from build123d import *

# Parameters (mm, degrees)
SKETCH1_R           = 1.75
SKETCH1_R_2         = 11.5
BOSS_EXTRUDE1_DEPTH = 3.2
BOSS_EXTRUDE2_START = 3.2
SKETCH1_5_R         = 2.55
SKETCH1_5_R_2       = 3
SKETCH1_5_R_3       = 11.5
SKETCH1_5_R_4       = 1.75
BOSS_EXTRUDE2_DEPTH = 3
BOSS_EXTRUDE3_START = 5
SKETCH1_6_R         = 2.55
BOSS_EXTRUDE3_DEPTH = 1.2
CUT_EXTRUDE2_START  = 3.2
SKETCH1_4_R         = 3
CUT_EXTRUDE2_DEPTH  = 3
FILLET1_R           = 3


with BuildPart() as part:
    # Sketch1 → Boss-Extrude1 (new body)
    with BuildSketch(Plane(origin=(0, -68.726755499, 0), x_dir=(1, 0, 0), z_dir=(0, 1, 0))):
        with BuildLine():
            Line((137.12924475, -27.521572875), (137.12924475, 3.821572875))
            ThreePointArc((137.12924475, 3.821572875), (136.992227909, 4.510403054), (136.602036956, 5.094365081))
            Line((136.602036956, 5.094365081), (133.273609831, 8.422792206))
            ThreePointArc((133.273609831, 8.422792206), (132.689647804, 8.812983159), (132.000817625, 8.95))
            Line((132.000817625, 8.95), (100.657671875, 8.95))
            ThreePointArc((100.657671875, 8.95), (99.968841697, 8.812983159), (99.384879669, 8.422792206))
            Line((99.384879669, 8.422792206), (96.056452544, 5.094365081))
            ThreePointArc((96.056452544, 5.094365081), (95.666261592, 4.510403054), (95.52924475, 3.821572875))
            Line((95.52924475, 3.821572875), (95.52924475, -27.521572875))
            ThreePointArc((95.52924475, -27.521572875), (95.666261592, -28.210403054), (96.056452544, -28.794365081))
            Line((96.056452544, -28.794365081), (99.384879669, -32.122792206))
            ThreePointArc((99.384879669, -32.122792206), (99.968841697, -32.512983159), (100.657671875, -32.65))
            Line((100.657671875, -32.65), (132.000817625, -32.65))
            ThreePointArc((132.000817625, -32.65), (132.689647804, -32.512983159), (133.273609831, -32.122792206))
            Line((133.273609831, -32.122792206), (136.602036956, -28.794365081))
            ThreePointArc((136.602036956, -28.794365081), (136.992227909, -28.210403054), (137.12924475, -27.521572875))
        make_face()
        with Locations((100.82924475, -27.35)):
            Circle(SKETCH1_R, mode=Mode.SUBTRACT)
        with Locations((100.82924475, 3.65)):
            Circle(SKETCH1_R, mode=Mode.SUBTRACT)
        with Locations((131.82924475, 3.65)):
            Circle(SKETCH1_R, mode=Mode.SUBTRACT)
        with Locations((131.82924475, -27.35)):
            Circle(SKETCH1_R, mode=Mode.SUBTRACT)
        with Locations((116.32924475, -11.85)):
            Circle(SKETCH1_R_2, mode=Mode.SUBTRACT)
    extrude(amount=BOSS_EXTRUDE1_DEPTH)

    # Sketch1<5> → Boss-Extrude2 (add)
    # profile 1 of 6: a face of its own
    with BuildSketch(Plane(origin=(0, -68.726755499, 0), x_dir=(1, 0, 0), z_dir=(0, 1, 0)).offset(BOSS_EXTRUDE2_START)):
        with BuildLine():
            ThreePointArc((133.273609831, -32.122792206), (132.689647804, -32.512983159), (132.000817625, -32.65))
            Line((132.000817625, -32.65), (156.32924475, -32.65))
            Line((156.32924475, -32.65), (156.32924475, 28))
            Line((156.32924475, 28), (116.32924475, 28))
            Line((116.32924475, 28), (116.32924475, 8.95))
            Line((116.32924475, 8.95), (132.000817625, 8.95))
            ThreePointArc((132.000817625, 8.95), (132.689647804, 8.812983159), (133.273609831, 8.422792206))
            Line((133.273609831, 8.422792206), (136.602036956, 5.094365081))
            ThreePointArc((136.602036956, 5.094365081), (136.992227909, 4.510403054), (137.12924475, 3.821572875))
            Line((137.12924475, 3.821572875), (137.12924475, -27.521572875))
            ThreePointArc((137.12924475, -27.521572875), (136.992227909, -28.210403054), (136.602036956, -28.794365081))
            Line((136.602036956, -28.794365081), (133.273609831, -32.122792206))
        make_face()
        with Locations((144.32924475, -16)):
            Circle(SKETCH1_5_R, mode=Mode.SUBTRACT)
        with Locations((152.32924475, -16)):
            Circle(SKETCH1_5_R, mode=Mode.SUBTRACT)
        with Locations((144.32924475, -8)):
            Circle(SKETCH1_5_R, mode=Mode.SUBTRACT)
        with Locations((152.32924475, -8)):
            Circle(SKETCH1_5_R, mode=Mode.SUBTRACT)
        with Locations((120.32924475, 16)):
            Circle(SKETCH1_5_R, mode=Mode.SUBTRACT)
        with Locations((120.32924475, 24)):
            Circle(SKETCH1_5_R, mode=Mode.SUBTRACT)
        with Locations((144.32924475, 0)):
            Circle(SKETCH1_5_R, mode=Mode.SUBTRACT)
        with Locations((152.32924475, 0)):
            Circle(SKETCH1_5_R, mode=Mode.SUBTRACT)
        with Locations((144.32924475, 8)):
            Circle(SKETCH1_5_R, mode=Mode.SUBTRACT)
        with Locations((152.32924475, 8)):
            Circle(SKETCH1_5_R, mode=Mode.SUBTRACT)
        with Locations((128.32924475, 16)):
            Circle(SKETCH1_5_R, mode=Mode.SUBTRACT)
        with Locations((136.32924475, 16)):
            Circle(SKETCH1_5_R, mode=Mode.SUBTRACT)
        with Locations((128.32924475, 24)):
            Circle(SKETCH1_5_R, mode=Mode.SUBTRACT)
        with Locations((136.32924475, 24)):
            Circle(SKETCH1_5_R, mode=Mode.SUBTRACT)
        with Locations((144.32924475, 16)):
            Circle(SKETCH1_5_R, mode=Mode.SUBTRACT)
        with Locations((152.32924475, 16)):
            Circle(SKETCH1_5_R, mode=Mode.SUBTRACT)
        with Locations((144.32924475, 24)):
            Circle(SKETCH1_5_R, mode=Mode.SUBTRACT)
        with Locations((152.32924475, 24)):
            Circle(SKETCH1_5_R, mode=Mode.SUBTRACT)
    # profile 2 of 6: a face of its own
    with BuildSketch(Plane(origin=(0, -68.726755499, 0), x_dir=(1, 0, 0), z_dir=(0, 1, 0)).offset(BOSS_EXTRUDE2_START)):
        with BuildLine():
            Line((100.657671875, -32.65), (132.000817625, -32.65))
            ThreePointArc((132.000817625, -32.65), (132.689647804, -32.512983159), (133.273609831, -32.122792206))
            Line((133.273609831, -32.122792206), (136.602036956, -28.794365081))
            ThreePointArc((136.602036956, -28.794365081), (136.992227909, -28.210403054), (137.12924475, -27.521572875))
            Line((137.12924475, -27.521572875), (137.12924475, 3.821572875))
            ThreePointArc((137.12924475, 3.821572875), (136.992227909, 4.510403054), (136.602036956, 5.094365081))
            Line((136.602036956, 5.094365081), (133.273609831, 8.422792206))
            ThreePointArc((133.273609831, 8.422792206), (132.689647804, 8.812983159), (132.000817625, 8.95))
            Line((132.000817625, 8.95), (116.32924475, 8.95))
            Line((116.32924475, 8.95), (100.657671875, 8.95))
            ThreePointArc((100.657671875, 8.95), (99.968841697, 8.812983159), (99.384879669, 8.422792206))
            Line((99.384879669, 8.422792206), (96.056452544, 5.094365081))
            ThreePointArc((96.056452544, 5.094365081), (95.666261592, 4.510403054), (95.52924475, 3.821572875))
            Line((95.52924475, 3.821572875), (95.52924475, -27.521572875))
            ThreePointArc((95.52924475, -27.521572875), (95.666261592, -28.210403054), (96.056452544, -28.794365081))
            Line((96.056452544, -28.794365081), (99.384879669, -32.122792206))
            ThreePointArc((99.384879669, -32.122792206), (99.968841697, -32.512983159), (100.657671875, -32.65))
        make_face()
        with Locations((100.82924475, -27.35)):
            Circle(SKETCH1_5_R_2, mode=Mode.SUBTRACT)
        with Locations((116.32924475, -11.85)):
            Circle(SKETCH1_5_R_3, mode=Mode.SUBTRACT)
        with Locations((131.82924475, -27.35)):
            Circle(SKETCH1_5_R_2, mode=Mode.SUBTRACT)
        with Locations((100.82924475, 3.65)):
            Circle(SKETCH1_5_R_2, mode=Mode.SUBTRACT)
        with Locations((131.82924475, 3.65)):
            Circle(SKETCH1_5_R_2, mode=Mode.SUBTRACT)
    # profile 3 of 6: a face of its own
    with BuildSketch(Plane(origin=(0, -68.726755499, 0), x_dir=(1, 0, 0), z_dir=(0, 1, 0)).offset(BOSS_EXTRUDE2_START)):
        with Locations((131.82924475, 3.65)):
            Circle(SKETCH1_5_R_2)
        with Locations((131.82924475, 3.65)):
            Circle(SKETCH1_5_R_4, mode=Mode.SUBTRACT)
    # profile 4 of 6: a face of its own
    with BuildSketch(Plane(origin=(0, -68.726755499, 0), x_dir=(1, 0, 0), z_dir=(0, 1, 0)).offset(BOSS_EXTRUDE2_START)):
        with Locations((131.82924475, -27.35)):
            Circle(SKETCH1_5_R_2)
        with Locations((131.82924475, -27.35)):
            Circle(SKETCH1_5_R_4, mode=Mode.SUBTRACT)
    # profile 5 of 6: a face of its own
    with BuildSketch(Plane(origin=(0, -68.726755499, 0), x_dir=(1, 0, 0), z_dir=(0, 1, 0)).offset(BOSS_EXTRUDE2_START)):
        with Locations((100.82924475, 3.65)):
            Circle(SKETCH1_5_R_2)
        with Locations((100.82924475, 3.65)):
            Circle(SKETCH1_5_R_4, mode=Mode.SUBTRACT)
    # profile 6 of 6: a face of its own
    with BuildSketch(Plane(origin=(0, -68.726755499, 0), x_dir=(1, 0, 0), z_dir=(0, 1, 0)).offset(BOSS_EXTRUDE2_START)):
        with Locations((100.82924475, -27.35)):
            Circle(SKETCH1_5_R_2)
        with Locations((100.82924475, -27.35)):
            Circle(SKETCH1_5_R_4, mode=Mode.SUBTRACT)
    extrude(amount=BOSS_EXTRUDE2_DEPTH)

    # Sketch1<6> → Boss-Extrude3 (add)
    with BuildSketch(Plane(origin=(0, -68.726755499, 0), x_dir=(1, 0, 0), z_dir=(0, 1, 0)).offset(BOSS_EXTRUDE3_START)):
        with Locations((152.32924475, -16)):
            Circle(SKETCH1_6_R)
        with Locations((144.32924475, -16)):
            Circle(SKETCH1_6_R)
        with Locations((144.32924475, -8)):
            Circle(SKETCH1_6_R)
        with Locations((152.32924475, -8)):
            Circle(SKETCH1_6_R)
        with Locations((152.32924475, 0)):
            Circle(SKETCH1_6_R)
        with Locations((144.32924475, 0)):
            Circle(SKETCH1_6_R)
        with Locations((152.32924475, 8)):
            Circle(SKETCH1_6_R)
        with Locations((152.32924475, 16)):
            Circle(SKETCH1_6_R)
        with Locations((144.32924475, 24)):
            Circle(SKETCH1_6_R)
        with Locations((152.32924475, 24)):
            Circle(SKETCH1_6_R)
        with Locations((136.32924475, 24)):
            Circle(SKETCH1_6_R)
        with Locations((136.32924475, 16)):
            Circle(SKETCH1_6_R)
        with Locations((128.32924475, 16)):
            Circle(SKETCH1_6_R)
        with Locations((128.32924475, 24)):
            Circle(SKETCH1_6_R)
        with Locations((120.32924475, 16)):
            Circle(SKETCH1_6_R)
        with Locations((120.32924475, 24)):
            Circle(SKETCH1_6_R)
        with Locations((144.32924475, 8)):
            Circle(SKETCH1_6_R)
        with Locations((144.32924475, 16)):
            Circle(SKETCH1_6_R)
    extrude(amount=BOSS_EXTRUDE3_DEPTH)

    # Sketch1<4> → Cut-Extrude2 (cut)
    with BuildSketch(Plane(origin=(0, -68.726755499, 0), x_dir=(1, 0, 0), z_dir=(0, 1, 0)).offset(CUT_EXTRUDE2_START)):
        with Locations((100.82924475, -27.35)):
            Circle(SKETCH1_4_R)
        with Locations((100.82924475, 3.65)):
            Circle(SKETCH1_4_R)
        with Locations((131.82924475, 3.65)):
            Circle(SKETCH1_4_R)
        with Locations((131.82924475, -27.35)):
            Circle(SKETCH1_4_R)
    extrude(amount=CUT_EXTRUDE2_DEPTH, mode=Mode.SUBTRACT)

    # Fillet1
    fillet1_edges = [part.edges().sort_by_distance(p)[0] for p in [
        (156.32924475, -64.026755499, 32.65),
        (156.32924475, -64.026755499, -28),
        (116.32924475, -64.026755499, -28),
        (116.32924475, -64.026755499, -8.95),
    ]]
    fillet(fillet1_edges, radius=FILLET1_R)


solid = part.part
Verification items for the finished model (mm, model axes). A direction names the side the tool comes from. Round coordinates to 2 decimals unless told otherwise and drop trailing zeros. Order: outer loops, then holes, each group sorted by start corner. A loop starts at its lowest first (then second) coordinate and runs counter-clockwise, first axis right, second up. Notation, with made-up numbers: (-31, 50) -> (-20, 50) arc R10 ccw to (-20, 57) -> close; hole circle Ø3 at (66, 3). An arc over 180 degrees is marked (long way). Put each result on its own line as item: value.
1) Mould release check, pull along X, two halves, no side actions. Record for faces 1 (the flat face through (134.961, -67.149, -6.735)), 2 (the cylindrical face through (141.78, -64.64, -0.11)), 3 (the flat face through (113, -66, -8.95)): +X half, -X half, draft (parallel to the pull), parting line (faces both ways), or undercut.
Final values:
face 1: +X half
face 2: undercut
face 3: draft
2) Section check A-A (z = 11.85). Record the cut outline in (x, y), then the cut area to 3 significant figures.
Final values:
outline: (95.53, -68.73) -> (104.83, -68.73) -> (104.83, -62.53) -> (95.53, -62.53) -> close; (127.83, -68.73) -> (137.13, -68.73) -> (137.13, -65.53) -> (156.33, -65.53) -> (156.33, -62.53) -> (127.83, -62.53) -> close
area: 173 mm^2
3) Set-up check for faces 4 (the flat face through (97.74, -65.67, -6.78)), 5 (the cylindrical face through (149.78, -64.64, -16.11)), 6 (the flat face through (102, -65.527, 29)): record each of +Z, -Z, +X, -X, +Y, -Y from which the full face is reachable in a straight line by a thin tool's end or side.
Final values:
face 4: -Z, -X, +Y, -Y
face 5: -Y
face 6: +Y
4) Material ranges on line 1 (Z direction, x = 132, y = -62.75); line 2 (X direction, y = -64.3, z = -3.65); line 3 (Z direction, x = 103, y = -65.25), recorded low to high.
Final values:
line 1: z = -28 to -6.65, -0.65 to 24.35, 30.35 to 32.65
line 2: x = 95.53 to 97.83, 103.83 to 128.83, 134.83 to 156.33
line 3: z = -8.95 to -5.72, -1.58 to 25.28, 29.42 to 32.65
5) Section check C-C (z = -16). Record the cut outline in (x, y), then the cut area to 3 significant figures.
Final values:
outline: (116.33, -65.53) -> (117.78, -65.53) -> (117.78, -63.73) -> (122.88, -63.73) -> (122.88, -65.53) -> (125.78, -65.53) -> (125.78, -63.73) -> (130.88, -63.73) -> (130.88, -65.53) -> (133.78, -65.53) -> (133.78, -63.73) -> (138.88, -63.73) -> (138.88, -65.53) -> (141.78, -65.53) -> (141.78, -63.73) -> (146.88, -63.73) -> (146.88, -65.53) -> (149.78, -65.53) -> (149.78, -63.73) -> (154.88, -63.73) -> (154.88, -65.53) -> (156.33, -65.53) -> (156.33, -62.53) -> (116.33, -62.53) -> close
area: 74.1 mm^2
6) Section check B-B (y = -67). Record the cut outline in (x, z), then the cut area to 3 significant figures.
Final values:
outline: (95.53, -3.82) arc R1.8 ccw to (96.06, -5.09) -> (99.38, -8.42) arc R1.8 ccw to (100.66, -8.95) -> (132, -8.95) arc R1.8 ccw to (133.27, -8.42) -> (136.6, -5.09) arc R1.8 ccw to (137.13, -3.82) -> (137.13, 27.52) arc R1.8 ccw to (136.6, 28.79) -> (133.27, 32.12) arc R1.8 ccw to (132, 32.65) -> (100.66, 32.65) arc R1.8 ccw to (99.38, 32.12) -> (96.06, 28.79) arc R1.8 ccw to (95.53, 27.52) -> close; hole circle Ø3.5 at (100.83, -3.65); hole circle Ø3.5 at (100.83, 27.35); hole circle Ø23 at (116.33, 11.85); hole circle Ø3.5 at (131.83, -3.65); hole circle Ø3.5 at (131.83, 27.35)
area: 1,240 mm^2
7) Section check D-D (z = 22.5). Record the cut outline in (x, y), then the cut area to 3 significant figures.
Final values:
outline: (95.53, -68.73) -> (111.99, -68.73) -> (111.99, -62.53) -> (95.53, -62.53) -> close; (120.67, -68.73) -> (137.13, -68.73) -> (137.13, -65.53) -> (156.33, -65.53) -> (156.33, -62.53) -> (120.67, -62.53) -> close
area: 262 mm^2
8) Depth check by flat-ended pin: pin 1 (2.5 mm diameter, centred on x = 153.5, z = 7, fed in from -Y); pin 2 (4 mm diameter, centred on x = 136.5, z = -16, fed in from -Y); pin 3 (3 mm diameter, centred on x = 133, z = -4.5, fed in from +Y). Enter the tip coordinate at first touch or a pass-through.
Final values:
pin 1: stops at y = -65.53
pin 2: stops at y = -63.73
pin 3: stops at y = -65.53
